Autodesk Inventor part; units mm, degrees
ref_plane "YZ Plane" through (0, 0, 0) normal (1, 0, 0) x (0, 1, 0)
ref_plane "XZ Plane" through (0, 0, 0) normal (0, 1, 0) x (-1, 0, 0)
ref_plane "XY Plane" through (0, 0, 0) normal (0, 0, 1) x (1, 0, 0)
sketch "Sketch1" plane through (0, 0, 0) normal (1, 0, 0) x (0, 1, 0)
  line L0 (1.2792, 416.4647) -> (-1.2608, 416.4647)
  line L1 (-1.2608, 416.4647) -> (-1.2608, -2.6353)
  line L2 (-1.2608, -2.6353) -> (1.2792, -2.6353)
  line L3 (1.2792, -2.6353) -> (1.2792, 416.4647)
  point P0 (0, 0)
  dimension "d0" = 2.54
  dimension "d1" = 419.1
extrude "Extrusion1" add sketch "Sketch1" along normal blind 330.2
sketch "Sketch2" plane through (0, -1.2608, -2.6353) normal (0, -1, 0) x (1, 0, 0)
  circle A0 centre (173.4912, 364.1066) radius 1.8317
  circle A1 centre (173.4912, 321.15) radius 1.8569
  circle A2 centre (125.7136, 321.15) radius 1.6798
  circle A3 centre (125.7136, 364.1066) radius 1.8317
  circle A4 centre (172.0099, 278.3905) radius 2.4145
  circle A5 centre (172.0099, 149.0149) radius 2.2543
  circle A6 centre (45.2863, 149.0149) radius 2.2807
  circle A7 centre (45.2863, 278.3905) radius 2.4145
  circle A8 centre (173.7693, 90.9127) radius 1.8262
  circle A9 centre (173.7693, 42.0819) radius 1.8081
  circle A10 centre (112.7456, 42.0819) radius 1.7821
  circle A11 centre (112.7456, 90.9127) radius 1.8323
  point P0 (0, 2.6353)
extrude "Extrusion2" cut sketch "Sketch2" against normal up to surface (2.54 mm away)
sketch "Sketch3" plane through (0, 1.2792, 416.4647) normal (0, 1, 0) x (1, 0, 0)
  line L0 (266.7, 209.1248) -> (266.7, 419.1) construction
  line L1 (0, 419.1) -> (330.2, 419.1)
  line L2 (266.7, 209.1248) -> (266.7, -0.8504) construction
  line L3 (330.2, 0) -> (330.2, 419.1)
  line L4 (330.2, 272.4308) -> (203.2, 272.4308)
  line L5 (203.2, 272.4308) -> (203.2, 145.4308)
  line L6 (203.2, 145.4308) -> (330.2, 145.4308)
  line L7 (330.2, 145.4308) -> (330.2, 272.4308)
  line L8 (330.2, 208.9308) -> (203.2, 208.9308) construction
  point P0 (0, 416.4647)
  dimension "d10" = 127
  dimension "d11" = 127
  dimension "d12" = 63.5
extrude "Extrusion4" cut sketch "Sketch3" against normal up to surface (2.54 mm away)
properties part number "Small Wall" material "Polycarbonate, Clear"
For this review, take the finished solid that the model builds, in its own axes (mm). Round coordinates to 2 decimals unless told otherwise and drop trailing zeros. Order: outer loops, then holes, each group sorted by start corner. A loop starts at its lowest first (then second) coordinate and runs counter-clockwise, first axis right, second up. Notation, with made-up numbers: M -8.5,-27.75 L 11.5,-27.75 A26 ccw 11.5,-5.75 Z; hole C 11.25,62.5 d10. An arc over 180 degrees is marked long. Write each question's results on one line, items separated by ' | '. Start each with the question number.
1. To check wall thickness, follow L1, parallel to Z at x = 311, y = 0.8; L2, parallel to X at y = 0.45, z = 262. State the ranges of each line that lie inside material, in increasing order. Write a range as [from, to].
2. Add section B-B (y = -0.7). State how many separate pieces and enclosed holes the cut face has, then the cut area to 3 significant figures.
3. Add section C-C (z = 223.5). State the section outline as (x, y) points, then the cut area to 3 significant figures.
4. Add section A-A (x = 237). State the section outline as (y, z) points.
5. Clearance check with a flat-ended pin moving along its axis: pin 1 Ø1.3 at (y, z) = (0.5, 190.5) entering from +X. State where the tip first meets the part, or that it passes through.
Output values:
1) L1: [-2.64, 144.03], [271.03, 416.46] | L2: [0, 203.2]
2) separate pieces: 1 | enclosed holes: 12 | area: 122,000 mm^2
3) outline: M 0,-1.26 L 203.2,-1.26 L 203.2,1.28 L 0,1.28 Z | area: 516 mm^2
4) outline: M -1.26,-2.64 L 1.28,-2.64 L 1.28,144.03 L -1.26,144.03 Z; M -1.26,271.03 L 1.28,271.03 L 1.28,416.46 L -1.26,416.46 Z
5) pin 1: x = 203.2
